Check sheet for the drawn part. Datum: minimum x, y, z corner. Units: mm. A direction names the side the tool comes from. Give positions to 0.01 mm unless a question says otherwise; leave off trailing zeros. Order: outer loops, then holes, each group sorted by start corner. A loop starts at its lowest first (then second) coordinate and runs counter-clockwise, first axis right, second up.
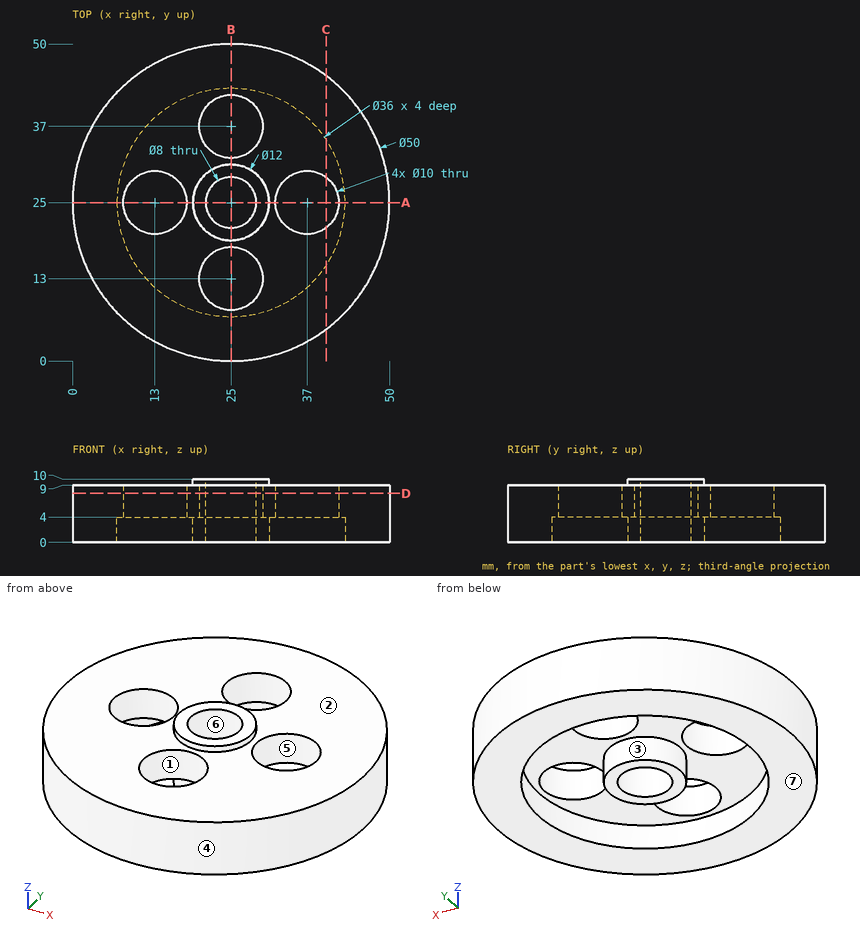
Item 1: Sectioned sample at C-C (x = 40). Enter the section's corners in (y, z), and give its area (3 significant figures).
Reported:
outline: (5, 0) - (15.05, 0) - (15.05, 4) - (21, 4) - (21, 9) - (5, 9) - close; (29, 4) - (34.95, 4) - (34.95, 0) - (45, 0) - (45, 9) - (29, 9) - close
area: 240 mm2
Item 2: Draft check along Y on the marked faces 4, 5, 6 and 7. Enter one of: released by +Y, released by -Y, zero draft, split by the parting line, or undercut.
Reported:
face 4: split by the parting line
face 5: undercut
face 6: undercut
face 7: zero draft
Item 3: Gauge pin test, flat ends, axial feed: pin 1 (2 mm diameter, centred on x = 32.5, y = 28.5, fed in from +Z); pin 2 (4 mm diameter, centred on y = 9, z = 1.5, fed in from -X); pin 3 (6 mm diameter, centred on y = 20, z = 5, fed in from -X); pin 4 (8 mm diameter, centred on x = 13, y = 25, fed in from +Z). Record the tip position at first contact, or that the pin passes through.
Reported:
pin 1: stops at z = 9
pin 2: stops at x = 4.29
pin 3: stops at x = 0.08
pin 4: passes through
Item 4: Sectioned sample at A-A (y = 25). Enter the section's corners in (x, z), and give its area (3 significant figures).
Reported:
outline: (0, 0) - (7, 0) - (7, 4) - (8, 4) - (8, 9) - (0, 9) - close; (18, 4) - (19, 4) - (19, 0) - (21, 0) - (21, 10) - (19, 10) - (19, 9) - (18, 9) - close; (29, 0) - (31, 0) - (31, 4) - (32, 4) - (32, 9) - (31, 9) - (31, 10) - (29, 10) - close; (42, 4) - (43, 4) - (43, 0) - (50, 0) - (50, 9) - (42, 9) - close
area: 186 mm2
Item 5: Set-up check for the marked faces 1, 2 and 3: record each of +Z, -Z, +X, -X, +Y, -Y from which the full face is reachable in a straight line by a thin tool's end or side.
Reported:
face 1: +Z, -Z
face 2: +Z
face 3: -Z
Item 6: Scan lines: L1, parallel to Y at x = 25, z = 8.25; L2, parallel to Y at x = 26, z = 7.75; L3, parallel to Z at x = 21, y = 44. Record each from-to range of solid material in increasing order.
Reported:
L1: y = 0 to 8, 18 to 21, 29 to 32, 42 to 50
L2: y = 0.02 to 8.1, 17.9 to 21.13, 28.87 to 32.1, 41.9 to 49.98
L3: z = 0 to 9
Item 7: Sectioned sample at D-D (z = 7.75). Enter the section's corners in (x, y), and give its area (3 significant figures).
Reported:
outline: circle Ø50 at (25, 25); hole circle Ø10 at (13, 25); hole circle Ø10 at (25, 13); hole circle Ø10 at (25, 37); hole circle Ø8 at (25, 25); hole circle Ø10 at (37, 25)
area: 1,600 mm2
